The listing builds one solid part. Answer for the finished solid, in the listing's coordinates (mm). Give positions to 0.01 mm unless a question says otherwise; leave off trailing zeros. Order: outer loops, then holes, each group sorted by start corner. A loop starts at its lowest first (then second) coordinate and runs counter-clockwise, first axis right, second up. Notation, with made-up numbers: M 28,-33.5 L 45,-33.5 A16 ccw 45,-5.5 Z; hole C -12,7 d1. An arc over 180 degrees is marked long. Answer as a JSON object with one key per item and string values. Group by question number.
Autodesk Inventor part; units mm, degrees
ref_plane "YZ Plane" through (0, 0, 0) normal (1, 0, 0) x (0, 1, 0)
ref_plane "XZ Plane" through (0, 0, 0) normal (0, 1, 0) x (-1, 0, 0)
ref_plane "XY Plane" through (0, 0, 0) normal (0, 0, 1) x (1, 0, 0)
sketch "Sketch1" plane through (0, 0, 0) normal (0, 0, 1) x (1, 0, 0)
  circle A0 centre (0, 0) radius 7.5
  dimension "d0" = 15
extrude "Extrusion1" add sketch "Sketch1" along normal blind 100
sketch "Sketch2" plane through (0, 0, 100) normal (0, 0, 1) x (1, 0, 0)
  circle A0 centre (0, 0) radius 4
  dimension "d3" = 8
extrude "Extrusion2" cut sketch "Sketch2" against normal blind 100
sketch "Sketch3" plane through (0, 0, 100) normal (0, 0, 1) x (1, 0, 0)
  circle A0 centre (0, 0) radius 7.5
extrude "Extrusion3" add sketch "Sketch3" along normal blind 400
sketch "Sketch4" plane through (0, 0, 500) normal (0, 0, 1) x (1, 0, 0)
  circle A0 centre (0, 0) radius 4
  dimension "d8" = 8
extrude "Extrusion4" cut sketch "Sketch4" against normal blind 400
sketch "Sketch5" plane through (0, 0, 500) normal (0, 0, 1) x (1, 0, 0)
  circle A0 centre (0, 0) radius 7.5
  dimension "d11" = 15
extrude "Extrusion5" cut sketch "Sketch5" against normal blind 50
thread "Thread1"
properties part number "ball pickr"
Item 1: Determine the mould class of faces 1 (the flat face through (3, -3, 0)), 2 (the cylindrical face through (-0.867, -3.905, 228.15)), 3 (the cylindrical face through (-7.493, -0.33, 221.85)) for opening direction X: released by +X, released by -X, zero draft, split by the parting line, or undercut.
Item 2: Consider probe 1 along Y at (x, z) = (0, 158.5); probe 2 along Y at (x, z) = (1, 334); probe 3 along X at (y, z) = (3, 67). Determine where each line is inside the solid, lowest interval first. Write a range as from..to.
Item 3: Section A-A (y = 0) is taken. Determine the outline of the cut face in (x, z).
Item 4: Flat-ended cylindrical pins translate along their axes: P1, Ø5, axis at x = 0, y = 0, coming from the -Z side; P2, Ø1.5, axis at x = 2.5, z = 63.5, coming from the -Y side. Find the tip coordinate at first contact, or state that the pin passes through.
Item 5: Section C-C (z = 363.5) is taken. Determine the outline of the cut face in (x, y).
Values found:
{
 "1": {"face 1": "zero draft", "face 2": "undercut", "face 3": "split by the parting line"},
 "2": {"probe 1": "y = -7.5..-4, 4..7.5", "probe 2": "y = -7.43..-3.87, 3.87..7.43", "probe 3": "x = -6.87..-2.65, 2.65..6.87"},
 "3": {"outline": "M -7.5,0 L -4,0 L -4,450 L -7.5,450 Z; M 4,0 L 7.5,0 L 7.5,450 L 4,450 Z"},
 "4": {"P1": "passes through", "P2": "stops at y = -7.29"},
 "5": {"outline": "C 0,0 d15; hole C 0,0 d8"}
}
